Model file for the job. Use its own axes, mm. Face numbers are marked on the shaded views. Round coordinates to 2 decimals unless told otherwise and drop trailing zeros. Loops run counter-clockwise (first coordinate to the right, second up) from the corner with the lowest first, then second, coordinate; pieces in that order, holes last. Notation, with made-up numbers: M 85.25,31.25 L 90.25,31.25 A5 cw 90.25,39.25 Z; hole C -32,57 d5. An arc over 180 degrees is marked long. Answer in a Markdown table with one row per item.
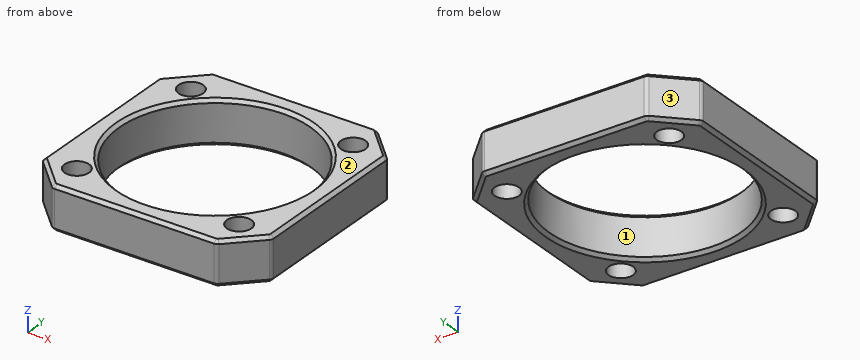
from build123d import *

# Parameters (mm, degrees)
SKETCH1_W            = 42
SKETCH1_H            = 42
SKETCH1_R            = 17.5
BOSS_EXTRUDE1_DEPTH  = 8
M4_CLEARANCE_HOLE1_D = 4.5
CIRPATTERN1_COUNT    = 4
CHAMFER2_SIZE        = 6
FILLET1_R            = 1
CHAMFER1_SIZE        = 0.6


with BuildPart() as part:
    # Sketch1 → Boss-Extrude1 (new body)
    with BuildSketch(Plane.XY):
        Rectangle(SKETCH1_W, SKETCH1_H)
        Circle(SKETCH1_R, mode=Mode.SUBTRACT)
    extrude(amount=BOSS_EXTRUDE1_DEPTH)

    # M4 Clearance Hole1 (through all)
    with Locations(Plane.XY.offset(8)):
        with Locations((14.849242405, 14.849242405)):
            m4_clearance_hole1 = Hole(M4_CLEARANCE_HOLE1_D / 2)

    # CirPattern1: M4 Clearance Hole1 ×4 about axis
    cirpattern1_axis = Axis((0, 0, 0), (0, 0, 1))
    for i in range(1, CIRPATTERN1_COUNT):
        add(m4_clearance_hole1.rotate(cirpattern1_axis, i * 360 / CIRPATTERN1_COUNT), mode=Mode.SUBTRACT)

    # Chamfer2
    chamfer2_edges = [part.edges().sort_by_distance(p)[0] for p in [
        (-21, 21, 4),
        (21, 21, 4),
        (21, -21, 4),
        (-21, -21, 4),
    ]]
    chamfer(chamfer2_edges, length=CHAMFER2_SIZE)

    # Fillet1
    fillet1_edges = [part.edges().sort_by_distance(p)[0] for p in [
        (-21, -15, 4),
        (-21, 15, 4),
        (15, 21, 4),
        (-15, 21, 4),
        (21, -15, 4),
        (21, 15, 4),
        (15, -21, 4),
        (-15, -21, 4),
    ]]
    fillet(fillet1_edges, radius=FILLET1_R)

    # Chamfer1
    chamfer1_edges = [part.edges().sort_by_distance(p)[0] for p in [
        (-17.5, 0, 0),
        (-17.5, 0, 8),
        (21, 0, 0),
        (21, 0, 8),
        (-21, 0, 0),
        (-18, 18, 0),
        (0, 21, 0),
        (18, 18, 0),
        (18, -18, 0),
        (0, -21, 0),
        (-18, -18, 0),
        (20.923879533, 14.96846987, 0),
        (14.96846987, 20.923879533, 0),
        (-14.96846987, 20.923879533, 0),
        (-20.923879533, 14.96846987, 0),
        (-20.923879533, -14.96846987, 0),
        (-14.96846987, -20.923879533, 0),
        (14.96846987, -20.923879533, 0),
        (20.923879533, -14.96846987, 0),
        (18, -18, 8),
        (0, 21, 8),
        (-18, 18, 8),
        (-21, 0, 8),
        (-18, -18, 8),
        (0, -21, 8),
        (18, 18, 8),
        (20.923879533, 14.96846987, 8),
        (14.96846987, 20.923879533, 8),
        (-14.96846987, 20.923879533, 8),
        (-20.923879533, 14.96846987, 8),
        (-20.923879533, -14.96846987, 8),
        (-14.96846987, -20.923879533, 8),
        (14.96846987, -20.923879533, 8),
        (20.923879533, -14.96846987, 8),
    ]]
    chamfer(chamfer1_edges, length=CHAMFER1_SIZE)


solid = part.part
1. Saw through at A-A (y = 0). Write the cut outline in (x, z).
Verdict:
| item | result |
|---|---|
| outline | M -21,0.6 L -20.4,0 L -18.1,0 L -17.5,0.6 L -17.5,7.4 L -18.1,8 L -20.4,8 L -21,7.4 Z; M 17.5,0.6 L 18.1,0 L 20.4,0 L 21,0.6 L 21,7.4 L 20.4,8 L 18.1,8 L 17.5,7.4 Z |
2. Mould opens along X. For the marked faces 1, 2 and 3 say: +X half, -X half, draft (parallel to the pull), parting line (faces both ways), or undercut.
Verdict:
| item | result |
|---|---|
| face 1 | undercut |
| face 2 | draft |
| face 3 | -X half |
3. Pin check, flat tips, straight feed: pin 1 (1.5 mm diameter, centred on y = -15.5, z = 5, fed in from +X); pin 2 (8 mm diameter, centred on x = 9.5, y = 5, fed in from +Z). Stop position of each tip, or through.
Verdict:
| item | result |
|---|---|
| pin 1 | stops at x = 20.99 |
| pin 2 | passes through |
4. Saw through at C-C (z = 3.5). Write the cut outline in (x, y).
Verdict:
| item | result |
|---|---|
| outline | M -21,-14.59 A1 ccw -20.71,-15.29 L -15.29,-20.71 A1 ccw -14.59,-21 L 14.59,-21 A1 ccw 15.29,-20.71 L 20.71,-15.29 A1 ccw 21,-14.59 L 21,14.59 A1 ccw 20.71,15.29 L 15.29,20.71 A1 ccw 14.59,21 L -14.59,21 A1 ccw -15.29,20.71 L -20.71,15.29 A1 ccw -21,14.59 Z; hole C 0,0 d35; hole C -14.85,-14.85 d4.5; hole C -14.85,14.85 d4.5; hole C 14.85,-14.85 d4.5; hole C 14.85,14.85 d4.5 |
5. Wall check: probe 1 along Y at (x, z) = (-8.5, 1); probe 2 along Y at (x, z) = (-14, 5.25); probe 3 along Y at (x, z) = (0, 5.5). Give the ranges that are in metal, low to high.
Verdict:
| item | result |
|---|---|
| probe 1 | y = -21 to -15.3, 15.3 to 21 |
| probe 2 | y = -21 to -16.93, -12.77 to -10.5, 10.5 to 12.77, 16.93 to 21 |
| probe 3 | y = -21 to -17.5, 17.5 to 21 |
6. Saw through at D-D (y = 16.5). State how many separate pieces and enclosed holes the cut face has, and give its area (3 significant figures).
Verdict:
| item | result |
|---|---|
| separate pieces | 4 |
| enclosed holes | 0 |
| area | 167 mm² |
